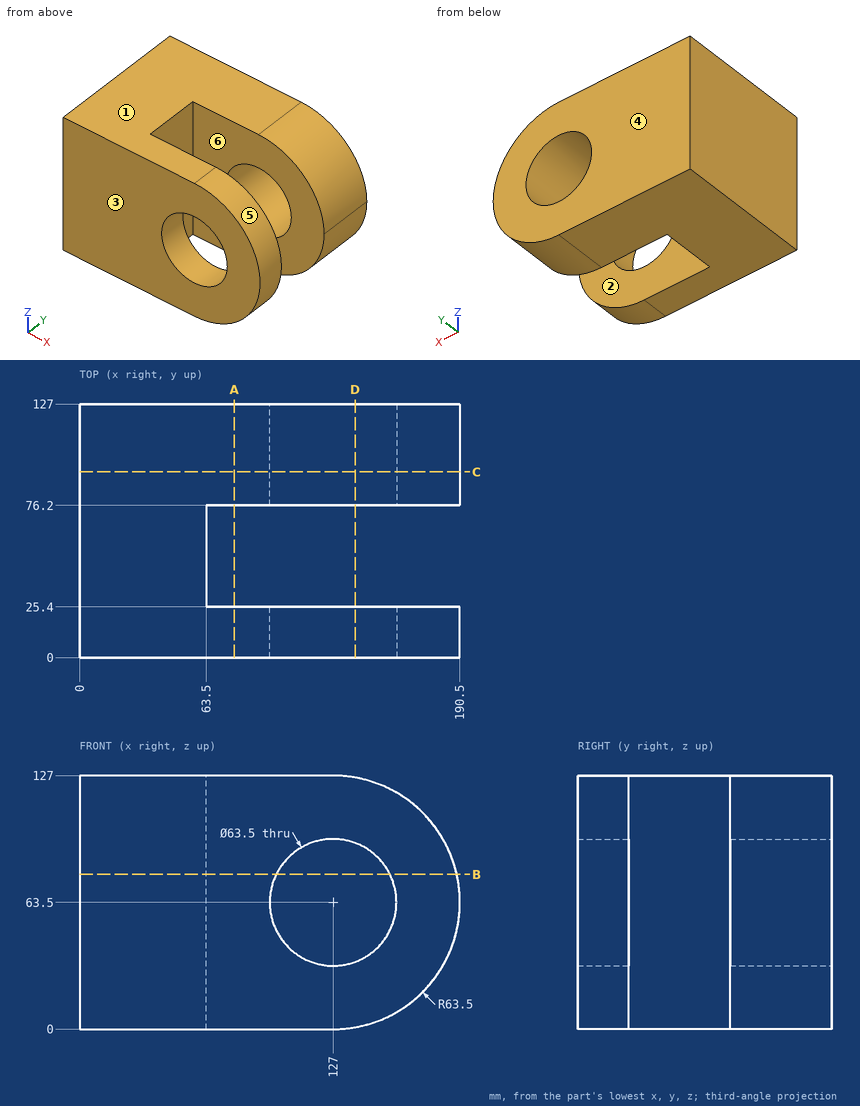
Here's the drawing with two shaded views (mm, measured from the low corner). I have some questions. A direction names the side the tool comes from. Coordinates: 2 decimals unless noted, no trailing zeros. Loops run counter-clockwise (first coordinate to the right, second up) from the corner with the lowest first, then second, coordinate; pieces in that order, holes last. Notation, with made-up numbers: (-36, 44) - (-16, 44) arc R5 ccw to (-16, 52) - close; hole circle Ø10 at (74.25, 60). An arc over 180 degrees is marked (long way). Answer as CSV lines item,"result". Start each with the question number.
1) Thinking about a two-plate mould opening in Y: for the marked faces 1, 2, 3 and 4, which applies, pulls with the +Y half, pulls with the -Y half, needs draft (parallel to the pull), parting line crosses it, or undercut?
2) For pin 1 (10 mm diameter, centred on y = 68, z = 28, fed in from +X); pin 2 (2 mm diameter, centred on y = 79.5, z = 53, fed in from +X), each with a flat end and sliding along its axis, tell me the tip position at first contact or that it passes through.
3) Suppose I cut it at A-A (x = 77.5). Please give me the cut outline in (y, z), plus the area to 3 significant figures.
4) Suppose I cut it at D-D (x = 138). Please give me the cut outline in (y, z).
5) Which directions (+Z, -Z, +X, -X, +Y, -Y) give clear straight access to the entire face, cutting with the end or side of a thin tool? Please do the marked faces 5 and 6.
6) Suppose I cut it at B-B (z = 77.5). Please give me the cut outline in (x, y).
7) Suppose I cut it at C-C (y = 93). Please give me the cut outline in (x, z).
8) I need wall thicknesses on line 1 (Y direction, x = 181.5, z = 84); line 2 (X direction, y = 6, z = 63); line 3 (X direction, y = 52.5, z = 45.5). Which ranges of each line are inside material? Lowest first, please. Write a range as from..to.
Check result:
1,face 1,"needs draft"
1,face 2,"undercut"
1,face 3,"pulls with the -Y half"
1,face 4,"pulls with the +Y half"
2,pin 1,"stops at x = 63.5"
2,pin 2,"stops at x = 189.79"
3,outline,"(0, 0) - (25.4, 0) - (25.4, 127) - (0, 127) - close; (76.2, 0) - (127, 0) - (127, 127) - (76.2, 127) - close"
3,area,"9,680 mm²"
4,outline,"(0, 0.96) - (25.4, 0.96) - (25.4, 33.72) - (0, 33.72) - close; (0, 93.28) - (25.4, 93.28) - (25.4, 126.04) - (0, 126.04) - close; (76.2, 0.96) - (127, 0.96) - (127, 33.72) - (76.2, 33.72) - close; (76.2, 93.28) - (127, 93.28) - (127, 126.04) - (76.2, 126.04) - close"
5,face 5,"+X, +Y, -Y"
5,face 6,"+Z, -Z, +X"
6,outline,"(0, 0) - (98.5, 0) - (98.5, 25.4) - (63.5, 25.4) - (63.5, 76.2) - (98.5, 76.2) - (98.5, 127) - (0, 127) - close; (155.5, 0) - (188.94, 0) - (188.94, 25.4) - (155.5, 25.4) - close; (155.5, 76.2) - (188.94, 76.2) - (188.94, 127) - (155.5, 127) - close"
7,outline,"(0, 0) - (127, 0) arc R63.5 ccw to (127, 127) - (0, 127) - close; hole circle Ø63.5 at (127, 63.5)"
8,line 1,"y = 0..25.4, 76.2..127"
8,line 2,"x = 0..95.25, 158.75..190.5"
8,line 3,"x = 0..63.5"
